Study the drawing (mm; zero at the part's minimum x, y, z) and answer. Round coordinates to 2 decimals unless told otherwise and drop trailing zeros. Loops run counter-clockwise (first coordinate to the right, second up) from the corner with the lowest first, then second, coordinate; pieces in that order, holes last. Notation, with made-up numbers: M 59,15 L 83,15 A14 cw 83,26 Z; hole C -35.5,13.5 d1. An arc over 180 degrees is marked long. Write each question's results on one line, items separated by ' | '.
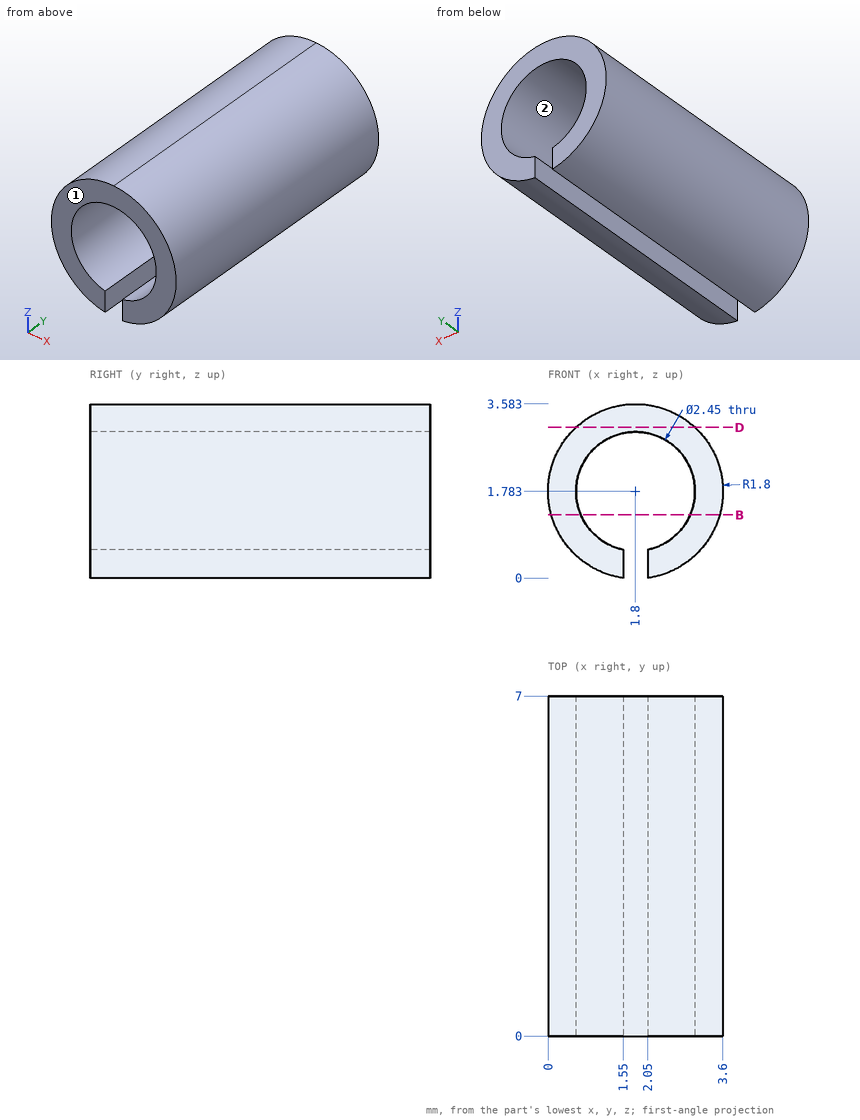
Item 1: The part is cut by section B-B (z = 1.3). Determine the outline of the cut face in (x, y) (1 decimal).
Outcome:
outline: M 0.1,0 L 0.7,0 L 0.7,7 L 0.1,7 Z; M 2.9,0 L 3.5,0 L 3.5,7 L 2.9,7 Z
Item 2: Flat-ended cylindrical pins translate along their axes: pin 1 (0.5 mm diameter, centred on y = 4, z = 0.5, fed in from -X) (1 decimal); pin 2 (0.5 mm diameter, centred on y = 4, z = 0.5, fed in from +X) (1 decimal). Find the tip coordinate at first contact, or state that the pin passes through.
Outcome:
pin 1: stops at x = 0.3 | pin 2: stops at x = 3.3
Item 3: The part is cut by section D-D (z = 3.1). Determine the outline of the cut face in (x, y), plus the area to 3 significant figures.
Outcome:
outline: M 0.57,0 L 3.03,0 L 3.03,7 L 0.57,7 Z | area: 17.2 mm2
Item 4: The mould has two halves that part along Z. Classify the marked faces 1 and 2: pulls with the +Z half, pulls with the -Z half, needs draft (parallel to the pull), parting line crosses it, or undercut.
Outcome:
face 1: needs draft | face 2: undercut
Item 5: Straight lines are drawn through the part: line 1 (Z direction, x = 1.8, y = 4.5); line 2 (Z direction, x = 2.8, y = 4.5) (1 decimal); line 3 (X direction, y = 0.5, z = 0.7) (1 decimal). For each, find the intervals that lie inside material, in ascending order.
Outcome:
line 1: z = 3.01 to 3.58 | line 2: z = 0.3 to 1.1, 2.5 to 3.3 | line 3: x = 0.4 to 1.2, 2.4 to 3.2
